Design review of the part built by this model. Coordinates are the model's own, in mm. A direction names the side the tool comes from. Give positions to 0.01 mm unless a question says otherwise; leave off trailing zeros. Order: outer loops, then holes, each group sorted by start corner. A loop starts at its lowest first (then second) coordinate and runs counter-clockwise, first axis right, second up. Notation, with made-up numbers: M -37.5,40 L 5.5,40 A12 ccw 5.5,47 Z; hole C 19,19.25 d6. An arc over 180 degrees is marked long. Answer as a JSON object with one key per item and string values.
from build123d import *

# Parameters (mm, degrees)
SKETCH1_W                   = 112.776
SKETCH1_H                   = 96.774
BOSS_EXTRUDE1_DEPTH         = 12.7
F_5_8_CLEARANCE_HOLE1_D     = 16.66875
F_5_8_CLEARANCE_HOLE1_DEPTH = 25.4
F_5_8_CLEARANCE_HOLE1_TIP   = 5.007797722
CUT_EXTRUDE2_START          = -12.7
SKETCH4_R                   = 11.509375
CUT_EXTRUDE2_DEPTH          = 12.7
CUT_EXTRUDE4_START          = 12.7
SKETCH5_R                   = 11.509375
CUT_EXTRUDE4_DEPTH          = 12.7
CUT_EXTRUDE6_START          = 12.7
SKETCH6_R                   = 16.6497
CUT_EXTRUDE6_DEPTH          = 2.8194
F_1_4_CLEARANCE_HOLE2_D     = 7.14375
F_1_4_CLEARANCE_HOLE2_DEPTH = 7.874
F_1_4_CLEARANCE_HOLE2_TIP   = 2.146199024
CUT_EXTRUDE8_START          = 12.7
SKETCH11_R                  = 3.175
CUT_EXTRUDE8_DEPTH          = 7.874


with BuildPart() as part:
    # Sketch1 → Boss-Extrude1 (new, symmetric)
    with BuildSketch(Plane(origin=(0, 0, 0), x_dir=(0, 1, 0), z_dir=(0, 0, 1))):
        Rectangle(SKETCH1_W, SKETCH1_H)
    extrude(amount=BOSS_EXTRUDE1_DEPTH, both=True)

    # 5/8 Clearance Hole1
    with Locations(Plane(origin=(0, 0, -12.7), x_dir=(-1, 0, 0), z_dir=(0, 0, -1))):
        with Locations((-32.512, -40.513), (-32.512, 40.513), (32.512, -40.513), (32.512, 40.513)):
            Hole(F_5_8_CLEARANCE_HOLE1_D / 2, depth=F_5_8_CLEARANCE_HOLE1_DEPTH)
            with Locations((0, 0, -(F_5_8_CLEARANCE_HOLE1_DEPTH + F_5_8_CLEARANCE_HOLE1_TIP / 2))):  # 118° drill point
                Cone(0, F_5_8_CLEARANCE_HOLE1_D / 2, F_5_8_CLEARANCE_HOLE1_TIP, mode=Mode.SUBTRACT)

    # Sketch4 → Cut-Extrude2 (cut)
    with BuildSketch(Plane(origin=(0, 0, 0), x_dir=(0, 1, 0), z_dir=(0, 0, 1)).offset(CUT_EXTRUDE2_START)):
        with Locations(Location((-27.813, 0, 0), (0, 0, 270))):
            Circle(SKETCH4_R)
        with Locations(Location((18.161, 0, 0), (0, 0, 270))):
            Circle(SKETCH4_R)
    extrude(amount=CUT_EXTRUDE2_DEPTH, mode=Mode.SUBTRACT)

    # Sketch5 → Cut-Extrude4 (cut)
    with BuildSketch(Plane(origin=(0, 0, 0), x_dir=(0, 1, 0), z_dir=(0, 0, 1)).offset(CUT_EXTRUDE4_START)):
        with Locations(Location((-18.161, 0, 0), (0, 0, 270))):
            Circle(SKETCH5_R)
        with Locations(Location((27.813, 0, 0), (0, 0, 270))):
            Circle(SKETCH5_R)
    extrude(amount=-CUT_EXTRUDE4_DEPTH, mode=Mode.SUBTRACT)

    # Sketch6 → Cut-Extrude6 (cut)
    with BuildSketch(Plane(origin=(0, 0, 0), x_dir=(0, 1, 0), z_dir=(0, 0, 1)).offset(CUT_EXTRUDE6_START)):
        with Locations(Location((-18.161, 0, 0), (0, 0, 270))):
            Circle(SKETCH6_R)
        with Locations(Location((27.813, 0, 0), (0, 0, 270))):
            Circle(SKETCH6_R)
    extrude(amount=-CUT_EXTRUDE6_DEPTH, mode=Mode.SUBTRACT)

    # 1/4 Clearance Hole2
    with Locations(Plane(origin=(0, 0, -12.7), x_dir=(-1, 0, 0), z_dir=(0, 0, -1))):
        with Locations((0, 49.149), (-32.512, 0.127)):
            Hole(F_1_4_CLEARANCE_HOLE2_D / 2, depth=F_1_4_CLEARANCE_HOLE2_DEPTH)
            with Locations((0, 0, -(F_1_4_CLEARANCE_HOLE2_DEPTH + F_1_4_CLEARANCE_HOLE2_TIP / 2))):  # 118° drill point
                Cone(0, F_1_4_CLEARANCE_HOLE2_D / 2, F_1_4_CLEARANCE_HOLE2_TIP, mode=Mode.SUBTRACT)

    # Sketch11 → Cut-Extrude8 (cut)
    with BuildSketch(Plane(origin=(0, 0, 0), x_dir=(0, 1, 0), z_dir=(0, 0, 1)).offset(CUT_EXTRUDE8_START)):
        with Locations(Location((-49.149, 0, 0), (0, 0, 270))):
            Circle(SKETCH11_R)
        with Locations(Location((-0.127, 32.512, 0), (0, 0, 270))):
            Circle(SKETCH11_R)
    extrude(amount=-CUT_EXTRUDE8_DEPTH, mode=Mode.SUBTRACT)


solid = part.part
(1) Tool access review of faces 4 (the flat face through (48.387, -1, 0)), 5 (the cylindrical face through (-0.46, 52.69, -8.71)), 6 (the flat face through (-33, 0, 4.826)): name each direction out of +Z, -Z, +X, -X, +Y, -Y from which nothing blocks a thin tool from reaching the whole face with its end or side.
Checked values:
{"face 4": "+Z, -Z, +X, +Y, -Y", "face 5": "-Z", "face 6": "+Z"}
(2) Draft analysis for pull direction X (two halves, no side actions). For faces 1 (the cylindrical face through (-33.597, 48.776, 0.178)), 2 (the flat face through (1, -56.388, 0)), 3 (the flat face through (-48.387, -1, 0)), state which applies: +X half, -X half, draft (parallel to the pull), parting line (faces both ways), or undercut.
Checked values:
{"face 1": "undercut", "face 2": "draft", "face 3": "-X half"}
(3) We need section B-B (x = -34). Write out the cut boundary in (y, z).
Checked values:
{"outline": "M -56.39,-12.7 L -48.71,-12.7 L -48.71,12.7 L -56.39,12.7 Z; M -32.31,-12.7 L 32.31,-12.7 L 32.31,12.7 L 2.68,12.7 L 2.68,4.83 L -2.93,4.83 L -2.93,12.7 L -32.31,12.7 Z; M 48.71,-12.7 L 56.39,-12.7 L 56.39,12.7 L 48.71,12.7 Z"}
(4) To check wall thickness, follow L1, parallel to Y at x = 0, z = 4.75; L2, parallel to Y at x = 0, z = -8; L3, parallel to X at y = 44.5, z = -0.25. State the ranges of each line that lie inside material, in increasing order. Write a range as from..to.
Checked values:
{"L1": "y = -56.39..-29.67, -6.65..16.3, 39.32..56.39", "L2": "y = -56.39..-39.32, -16.3..6.65, 29.67..45.58, 52.72..56.39", "L3": "x = -48.39..-39.83, -25.19..25.19, 39.83..48.39"}
(5) We need section A-A (y = -37.5). Write out the cut boundary in (x, z), plus the area to 3 significant figures.
Checked values:
{"outline": "M -48.39,-12.7 L -40.28,-12.7 L -40.28,12.7 L -48.39,12.7 Z; M -24.74,-12.7 L -6.22,-12.7 L -6.22,0 L 6.22,0 L 6.22,-12.7 L 24.74,-12.7 L 24.74,12.7 L -24.74,12.7 Z; M 40.28,-12.7 L 48.39,-12.7 L 48.39,12.7 L 40.28,12.7 Z", "area": "1,510 mm^2"}
(6) Insertion check: pin 1 (14 mm diameter, centred on x = 0, y = -18.161, fed in from +Z). The pin has a flat end and moves straight along its axis. Give the tip position at first contact, or say it passes through.
Checked values:
{"pin 1": "stops at z = 0"}
(7) We need section C-C (y = 21.5). Write out the cut boundary in (x, z).
Checked values:
{"outline": "M -48.39,-12.7 L -11.01,-12.7 L -11.01,0 L -9.62,0 L -9.62,9.88 L -15.41,9.88 L -15.41,12.7 L -48.39,12.7 Z; M 9.62,0 L 11.01,0 L 11.01,-12.7 L 48.39,-12.7 L 48.39,12.7 L 15.41,12.7 L 15.41,9.88 L 9.62,9.88 Z"}
(8) We need section D-D (y = -12.5). Write out the cut boundary in (x, z).
Checked values:
{"outline": "M -48.39,-12.7 L 48.39,-12.7 L 48.39,12.7 L 15.66,12.7 L 15.66,9.88 L 10.02,9.88 L 10.02,0 L -10.02,0 L -10.02,9.88 L -15.66,9.88 L -15.66,12.7 L -48.39,12.7 Z"}
